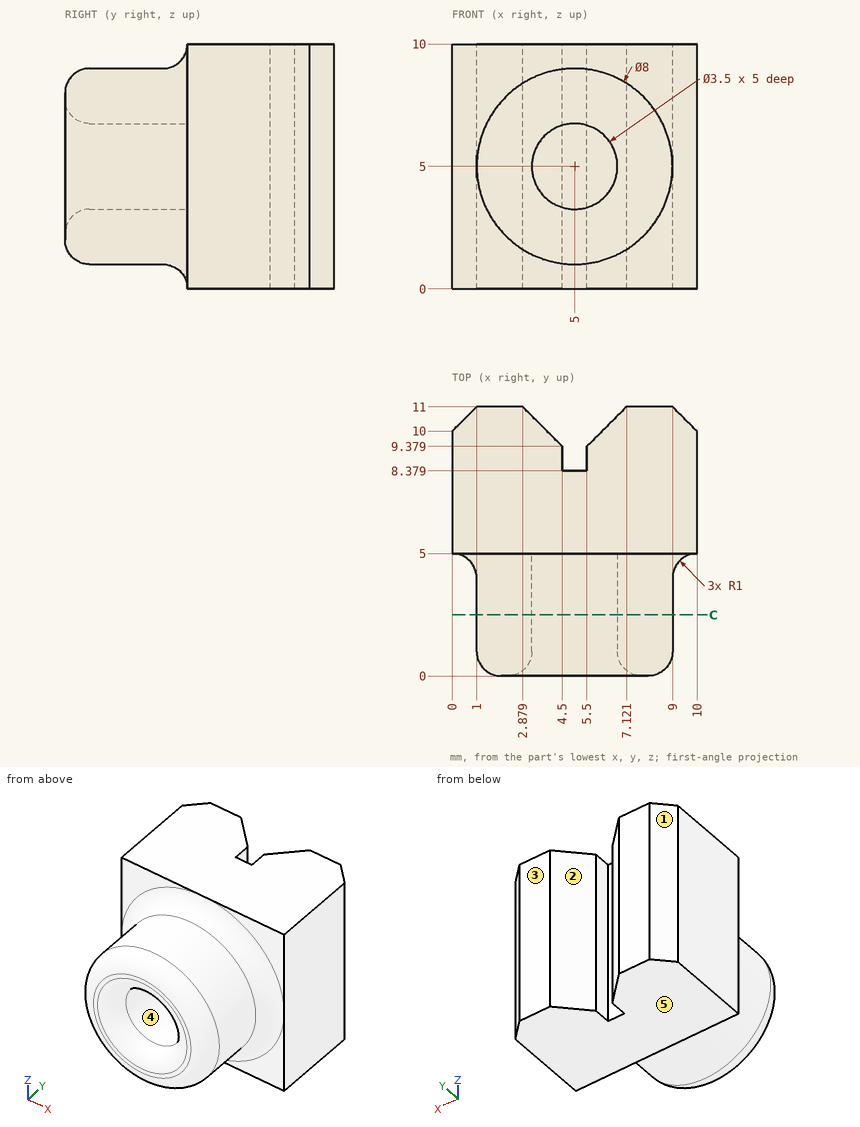
Print and shaded views of the part. All mm, measured from the part's lowest x, y and z. A direction names the side the tool comes from. Coordinates: 2 decimals unless noted, no trailing zeros. Order: outer loops, then holes, each group sorted by start corner. A loop starts at its lowest first (then second) coordinate and runs counter-clockwise, first axis right, second up. Notation, with made-up numbers: M -5,-8.5 L 2,-8.5 A15 ccw 2,-3.5 Z; hole C 75,47.5 d10. An arc over 180 degrees is marked long. Answer as CSV lines item,"result".
1) Flat gauge pins, fed straight in: P1, Ø0.8, axis at x = 5, z = 4.5, coming from the +Y side; P2, Ø1, axis at y = 1.5, z = 6.5, coming from the +X side; P3, Ø3, axis at x = 2.5, y = 2, coming from the -Z side. Where does each tip first touch, or does it go through?
Verdict:
P1,"y = 8.38"
P2,"x = 8.87"
P3,"z = 1.13"
2) 3-axis set-ups, long thin cutter, end or side, ignore diameter. For the marked faces 4 and 5: which of +Z, -Z, +X, -X, +Y, -Y reach the whole face in a straight line?
Verdict:
face 4,"-Y"
face 5,"-Z, +X, -X, +Y, -Y"
3) Mould opens along X. For the marked faces 1, 2 and 3 say: released by +X, released by -X, zero draft, split by the parting line, or undercut.
Verdict:
face 1,"released by -X"
face 2,"undercut"
face 3,"zero draft"
4) Cut at C-C (y = 2.5). List the corners of the cut face in (x, z).
Verdict:
outline,"C 5,5 d8; hole C 5,5 d3.5"
5) Drill centre lines: L1, parallel to Z at x = 5, y = 2.4; L2, parallel to Y at x = 5, z = 7.75; L3, parallel to X at y = 9.75, z = 3.5. Where is each one in solid material? Low to high. Write a range as from..to.
Verdict:
L1,"1..3.25, 6.75..9"
L2,"0..8.38"
L3,"0..4.13, 5.87..10"
